Build history of the part. All positions in model axes, mm. A direction names the side the tool comes from. Round coordinates to 2 decimals unless told otherwise and drop trailing zeros. Write each loop counter-clockwise with the first axis right and the second up, starting at its lowest first coordinate (ties: lowest second). Pieces come first, ordered by that corner, then holes. Notation, with made-up numbers: M -7.5,86.25 L 40.5,86.25 A17 cw 40.5,98.25 Z; hole C -15,55 d1. An arc over 180 degrees is marked long. One line per item, written item: value. Start each with the question number.
```python
from build123d import *

# Parameters (mm, degrees)
CROQUIS1_W              = 179.6
CROQUIS1_H              = 119.6
CROQUIS1_W_2            = 176.4
CROQUIS1_H_2            = 116.4
SALIENTE_EXTRUIR1_DEPTH = 40
CROQUIS2_W              = 196.4
CROQUIS2_H              = 136.4
CROQUIS2_W_2            = 176.4
CROQUIS2_H_2            = 116.4
SALIENTE_EXTRUIR2_DEPTH = 4
CROQUIS10_W             = 179.6
CROQUIS10_H             = 119.6
CORTAR_EXTRUIR6_DEPTH   = 128.398901094
CROQUIS7_R              = 1.6
CORTAR_EXTRUIR3_DEPTH   = 120.626418487
CORTAR_EXTRUIR5_START   = -1
CORTAR_EXTRUIR5_DEPTH   = 119.626418487
REDONDEO1_R             = 5
CHAFL_N2_SIZE           = 0.5
CHAFL_N3_SIZE           = 1


with BuildPart() as part:
    # Croquis1 → Saliente-Extruir1 (new body)
    with BuildSketch(Plane.XY):
        Rectangle(CROQUIS1_W, CROQUIS1_H)
        Rectangle(CROQUIS1_W_2, CROQUIS1_H_2, mode=Mode.SUBTRACT)
    extrude(amount=SALIENTE_EXTRUIR1_DEPTH)

    # Croquis2 → Saliente-Extruir2 (add)
    with BuildSketch(Plane(origin=(0, 0, 0), x_dir=(-1, 0, 0), z_dir=(0, 0, -1))):
        Rectangle(CROQUIS2_W, CROQUIS2_H)
        Rectangle(CROQUIS2_W_2, CROQUIS2_H_2, mode=Mode.SUBTRACT)
    extrude(amount=SALIENTE_EXTRUIR2_DEPTH)

    # Croquis10 → Cortar-Extruir6 (cut, through all)
    with BuildSketch(Plane.XY.offset(40)):
        Rectangle(CROQUIS10_W, CROQUIS10_H)
    extrude(amount=-CORTAR_EXTRUIR6_DEPTH, mode=Mode.SUBTRACT)

    # Croquis7 → Cortar-Extruir3 (cut, through all)
    with BuildSketch(Plane(origin=(0, 0, -4), x_dir=(-1, 0, 0), z_dir=(0, 0, -1))):
        with Locations((0, 63.2)):
            Circle(CROQUIS7_R)
        with Locations((93.2, 63.2)):
            Circle(CROQUIS7_R)
        with Locations(Location((-93.2, 63.2, 0), (0, 0, 180))):
            Circle(CROQUIS7_R)
        with Locations((-93.2, -63.2)):
            Circle(CROQUIS7_R)
        with Locations(Location((93.2, -63.2, 0), (0, 0, 180))):
            Circle(CROQUIS7_R)
        with Locations(Location((0, -63.2, 0), (0, 0, 180))):
            Circle(CROQUIS7_R)
    extrude(amount=-CORTAR_EXTRUIR3_DEPTH, mode=Mode.SUBTRACT)

    # Croquis9 → Cortar-Extruir5 (cut, through all)
    with BuildSketch(Plane(origin=(0, 0, -4), x_dir=(-1, 0, 0), z_dir=(0, 0, -1)).offset(CORTAR_EXTRUIR5_START)):
        Polygon((-90.024573519, 63.2), (-91.61228676, 65.95), (-94.78771324, 65.95), (-96.375426481, 63.2), (-94.78771324, 60.45), (-91.61228676, 60.45), align=None)
        Polygon((3.175426481, 63.2), (1.58771324, 65.95), (-1.58771324, 65.95), (-3.175426481, 63.2), (-1.58771324, 60.45), (1.58771324, 60.45), align=None)
        Polygon((3.175426481, -63.2), (1.58771324, -60.45), (-1.58771324, -60.45), (-3.175426481, -63.2), (-1.58771324, -65.95), (1.58771324, -65.95), align=None)
        Polygon((-90.024573519, -63.2), (-91.61228676, -60.45), (-94.78771324, -60.45), (-96.375426481, -63.2), (-94.78771324, -65.95), (-91.61228676, -65.95), align=None)
        Polygon((96.375426481, -63.2), (94.78771324, -60.45), (91.61228676, -60.45), (90.024573519, -63.2), (91.61228676, -65.95), (94.78771324, -65.95), align=None)
        Polygon((96.375426481, 63.2), (94.78771324, 65.95), (91.61228676, 65.95), (90.024573519, 63.2), (91.61228676, 60.45), (94.78771324, 60.45), align=None)
    extrude(amount=-CORTAR_EXTRUIR5_DEPTH, mode=Mode.SUBTRACT)

    # Redondeo1
    redondeo1_edges = [part.edges().sort_by_distance(p)[0] for p in [
        (-98.2, -68.2, -2),
        (-98.2, 68.2, -2),
        (98.2, 68.2, -2),
        (98.2, -68.2, -2),
    ]]
    fillet(redondeo1_edges, radius=REDONDEO1_R)

    # Chaflán2
    chafl_n2_edges = [part.edges().sort_by_distance(p)[0] for p in [
        (98.2, 0, 0),
        (-98.2, 0, 0),
        (0, -68.2, 0),
        (0, 68.2, 0),
        (-96.735533906, 66.735533906, 0),
        (-96.735533906, -66.735533906, 0),
        (96.735533906, -66.735533906, 0),
        (96.735533906, 66.735533906, 0),
    ]]
    chamfer(chafl_n2_edges, length=CHAFL_N2_SIZE)

    # Chaflán3
    chafl_n3_edges = [part.edges().sort_by_distance(p)[0] for p in [
        (-91.6, 63.2, -4),
        (91.6, 63.2, -4),
        (94.8, -63.2, -4),
        (-94.8, -63.2, -4),
        (-1.6, -63.2, -4),
        (1.6, 63.2, -4),
    ]]
    chamfer(chafl_n3_edges, length=CHAFL_N3_SIZE - 0.0001)  # a hair under: the kernel refuses the full size


solid = part.part
```
Item 1: Cut at B-B, the plane x = -59.5. Write the cut outline in (y, z).
Item 2: Cut at C-C, the plane z = -1.4. Count the separate pieces of the cut face and the enclosed holes in it, plus the area to 3 significant figures.
Item 3: Cut at A-A, the plane y = 33. Write the cut outline in (x, z), plus the area to 4 significant figures.
Item 4: Drop flat-ended pins along their axis: pin 1 (1.6 mm diameter, centred on x = -0.5, y = -64, fed in from +Z); pin 2 (5 mm diameter, centred on x = -93.2, y = 63.2, fed in from -Z). Give the stop position or say it passes through.
Item 5: Drill centre lines: line 1 (X direction, y = -63.2, z = -2.95); line 2 (Y direction, x = 0, z = -2.95); line 3 (Y direction, x = -93.2, z = -2.95). Where is each one in solid material? Low to high.
Item 6: Which spindle directions (+Z, -Z, +X, -X, +Y, -Y) get a long thin tool onto all of the face, cutting with end or side? Do faces 5 (the flat face through (0, -60, -4)), 6 (the flat face through (-1, -59.8, -2)), 7 (the flat face through (91.8, 64.5, -3)). Say none if no direction does.
Item 7: Two-plate mould, pull along Y, no slides. Class faces 1 (the flat face through (89.8, -1, -2)), 2 (the conical face through (96.441, -66.514, -0.135)), 3 (the conical face through (-96.441, 66.514, -0.135)), 4 (the flat face through (-1.4, 64.5, -3)): pulls with the +Y half, pulls with the -Y half, needs draft (parallel to the pull), parting line crosses it, or undercut.
Computed values:
1. outline: M -68.2,-4 L -59.8,-4 L -59.8,0 L -67.7,0 L -68.2,-0.5 Z; M 59.8,-4 L 68.2,-4 L 68.2,-0.5 L 67.7,0 L 59.8,0 Z
2. separate pieces: 1
2. enclosed holes: 7
2. area: 5,130 mm2
3. outline: M -98.2,-4 L -89.8,-4 L -89.8,0 L -97.7,0 L -98.2,-0.5 Z; M 89.8,-4 L 98.2,-4 L 98.2,-0.5 L 97.7,0 L 89.8,0 Z
3. area: 66.95 mm2
4. pin 1: stops at z = -3
4. pin 2: stops at z = -3.9
5. line 1: x = -98.2 to -96.38, -90.02 to -3.18, 3.18 to 90.02, 96.38 to 98.2
5. line 2: y = -68.2 to -65.95, -60.45 to -59.8, 59.8 to 60.45, 65.95 to 68.2
5. line 3: y = -68.2 to -65.95, -60.45 to 60.45, 65.95 to 68.2
6. face 5: -Z, +X, -X, +Y, -Y
6. face 6: +Z, -Z
6. face 7: +Z
7. face 1: undercut
7. face 2: pulls with the -Y half
7. face 3: pulls with the +Y half
7. face 4: undercut
